Job drawing, mm, ordinate dimensions from the low corner. One solid piece. A direction names the side the tool comes from. Give positions to 0.01 mm unless a question says otherwise; leave off trailing zeros. Write each loop counter-clockwise with the first axis right and the second up, starting at its lowest first coordinate (ties: lowest second). Pieces come first, ordered by that corner, then holes. Notation, with made-up numbers: (65, 41) - (111, 41) arc R18 cw to (111, 70) - close; hole circle Ø10 at (45.25, 63). An arc over 180 degrees is marked (long way). Answer as a JSON object with one key per item and string values.
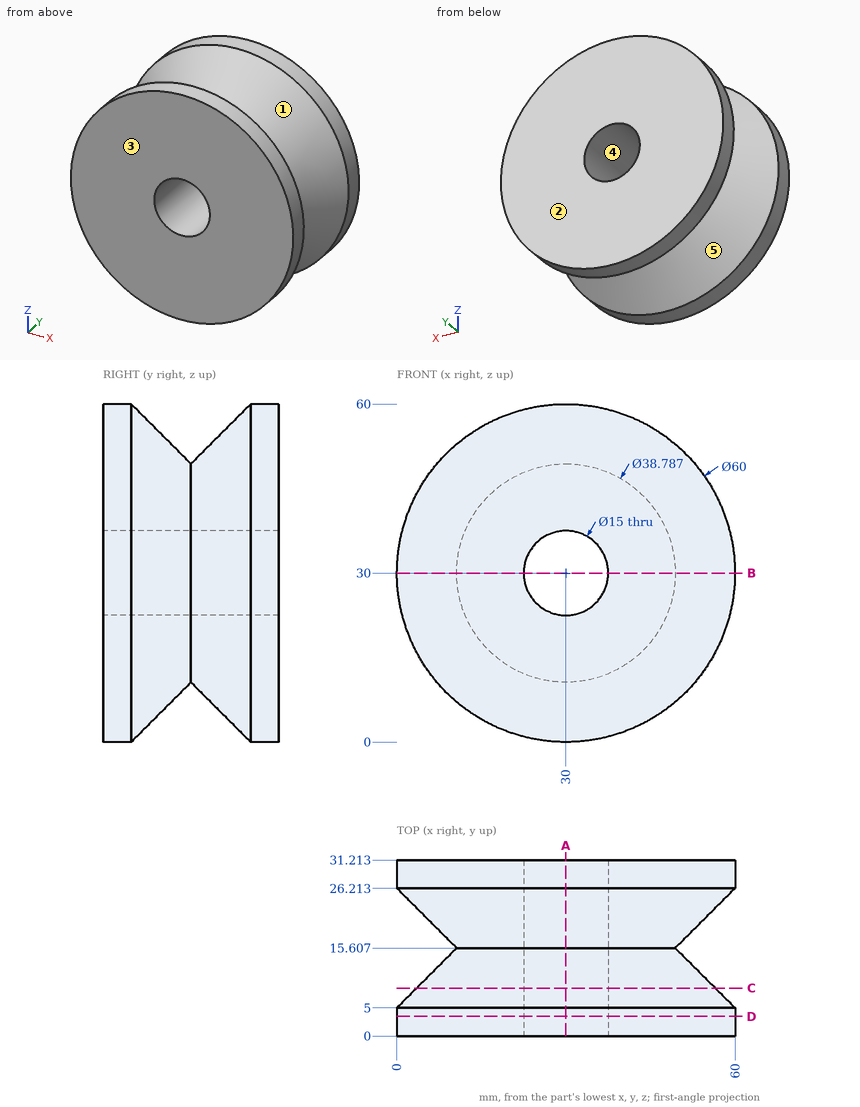
Item 1: Which spindle directions (+Z, -Z, +X, -X, +Y, -Y) get a long thin tool onto all of the face, cutting with end or side? Do the marked faces 1 and 2. Say none if no direction does.
Entries:
{"face 1": "none", "face 2": "+Z, -Z, +X, -X, +Y"}
Item 2: Cut at D-D (y = 3.5). Give the cut face in (x, z).
Entries:
{"outline": "circle Ø60 at (30, 30); hole circle Ø15 at (30, 30)"}
Item 3: Flat gauge pins, fed straight in: P1, Ø1.5, axis at x = 41.5, y = 16, coming from the +Z side (1 decimal); P2, Ø10, axis at x = 53, y = 9.5, coming from the +Z side (1 decimal); P3, Ø4, axis at x = 12, y = 8, coming from the -Z side (1 decimal). Where does each tip first touch, or does it go through?
Entries:
{"P1": "z = 47.1", "P2": "z = 51.7", "P3": "z = 6.8"}
Item 4: Mould opens along Z. For the marked faces 3, 4 and 5 say: +Z half, -Z half, draft (parallel to the pull), parting line (faces both ways), or undercut.
Entries:
{"face 3": "draft", "face 4": "undercut", "face 5": "parting line"}
Item 5: Cut at C-C (y = 8.5). Give the cut face in (x, z), and give its area (3 significant figures).
Entries:
{"outline": "circle Ø53 at (30, 30); hole circle Ø15 at (30, 30)", "area": "2,030 mm2"}
Item 6: Cut at B-B (z = 30). Give the cut face in (x, y), and give its area (3 significant figures).
Entries:
{"outline": "(0, 0) - (22.5, 0) - (22.5, 31.21) - (0, 31.21) - (0, 26.21) - (10.61, 15.61) - (0, 5) - close; (37.5, 0) - (60, 0) - (60, 5) - (49.39, 15.61) - (60, 26.21) - (60, 31.21) - (37.5, 31.21) - close", "area": "1,180 mm2"}
Item 7: Probe line 1 (Z direction, x = 30, y = 14); line 2 (Y direction, x = 51, z = 41.5) (1 decimal); line 3 (Z direction, x = 30, y = 19) (1 decimal). List the from-to ranges inside material, lowest first. Write a range as from..to.
Entries:
{"line 1": "9..22.5, 37.5..51", "line 2": "0..11.1, 20.2..31.2", "line 3": "7.2..22.5, 37.5..52.8"}
Item 8: Cut at A-A (x = 30). Give the cut face in (y, z), and give its area (3 significant figures).
Entries:
{"outline": "(0, 0) - (5, 0) - (15.61, 10.61) - (26.21, 0) - (31.21, 0) - (31.21, 22.5) - (0, 22.5) - close; (0, 37.5) - (31.21, 37.5) - (31.21, 60) - (26.21, 60) - (15.61, 49.39) - (5, 60) - (0, 60) - close", "area": "1,180 mm2"}
